Read the model definition and answer for the solid it produces. Units are mm, in the model's axes. Face numbers are marked on the shaded views. Round coordinates to 2 decimals unless told otherwise and drop trailing zeros. Loops run counter-clockwise (first coordinate to the right, second up) from the corner with the lowest first, then second, coordinate; pieces in that order, holes last. Notation, with made-up numbers: (12.25, 83.5) - (45.25, 83.5) arc R11 ccw to (45.25, 92.5) - close; hole circle Ø2 at (56, 24.5). An arc over 180 degrees is marked (long way). Use CSV: the item, a comma, the result in double quotes. Start each with the question number.
1. Find section C-C (z = 21.25). Give the vertices of the cut face in (x, y), and give its area (3 significant figures).
2. Consider line 1 along Y through (x, z) = (0, 22.75); line 2 along X through (y, z) = (1.25, 28.25). Determine where each line is inside the solid, lowest interval first.
3. Determine the mould class of the marked faces 1, 2 and 3 for opening direction X: +X half, -X half, draft (parallel to the pull), parting line (faces both ways), or undercut.
4. Find section A-A (y = 0). Give the vertices of the cut face in (x, z), and give its area (3 significant figures).
5. Find section D-D (z = 17). Give the vertices of the cut face in (x, y).
6. Given pin 1 Ø1 at (y, z) = (-1, 6.5) entering from +X; pin 2 Ø5 at (x, z) = (-0.5, 16.5) entering from +Y; pin 3 Ø2 at (x, z) = (-1.5, 15.5) entering from +Y, each flat-ended and moving along its own axis, determine where each tip first touches the part or whether it passes through.
from build123d import *

# Parameters (mm, degrees)
SKETCH1_R           = 4.5
SKETCH1_R_2         = 2.5
BOSS_EXTRUDE1_DEPTH = 2
SKETCH5_R           = 2.5
BOSS_EXTRUDE3_DEPTH = 28
SKETCH6_R           = 1.5
CUT_EXTRUDE3_DEPTH  = 10
BOSS_EXTRUDE4_START = 1
SKETCH7_R           = 2.5
BOSS_EXTRUDE4_DEPTH = 1
FILLET1_R           = 2


with BuildPart() as part:
    # Sketch1 → Boss-Extrude1 (new body)
    with BuildSketch(Plane.XY):
        Circle(SKETCH1_R)
        Circle(SKETCH1_R_2, mode=Mode.SUBTRACT)
    extrude(amount=BOSS_EXTRUDE1_DEPTH)



with BuildPart() as body_2:
    # Sketch5 → Boss-Extrude3 (new body)
    with BuildSketch(Plane.XY.offset(2)):
        Circle(SKETCH5_R)
    extrude(amount=BOSS_EXTRUDE3_DEPTH)

    # Sketch6 → Cut-Extrude3 (cut)
    with BuildSketch(Plane.XY.offset(30)):
        Circle(SKETCH6_R)
    extrude(amount=-CUT_EXTRUDE3_DEPTH, mode=Mode.SUBTRACT)


with BuildPart() as part_1:
    add(part.part)

    add(body_2.part)  # Boss-Extrude4 merges body 2
    # Sketch7 → Boss-Extrude4 (add)
    with BuildSketch(Plane(origin=(0, 0, 2), x_dir=(-1, 0, 0), z_dir=(0, 0, -1)).offset(BOSS_EXTRUDE4_START)):
        Circle(SKETCH7_R)
    extrude(amount=-BOSS_EXTRUDE4_DEPTH)

    # Fillet1
    # the kernel refuses this fillet: 2 mm, written as the material it takes off along each edge
    with BuildSketch(Plane(origin=(0, 0, 0), x_dir=(1, 0, 0), z_dir=(0, -1, 0))) as fillet1_piece_1:
        with BuildLine():
            CenterArc((4.232050808, 2), FILLET1_R, 210, 60)
            Line((2.5, 1), (2.465358984, 0.98))
            ThreePointArc((2.465358984, 0.98), (2.46, 0.5), (2.46, 0))
            Line((2.46, 0), (2.5, -0.04))
            Line((2.5, -0.04), (4.232050808, -0.04))
            Line((4.232050808, -0.04), (4.232050808, 0))
        make_face()
    revolve(axis=Axis((0, 0, 0), (0, 0, 1)), mode=Mode.SUBTRACT)


solid = part_1.part
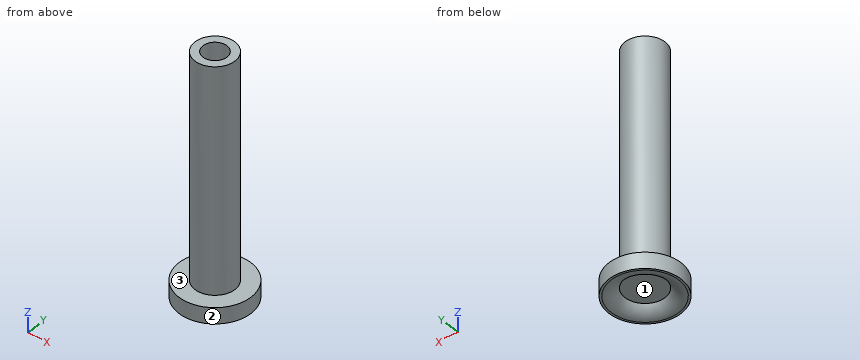
Filled sheet:
1,outline,"circle Ø5 at (0, 0); hole circle Ø3 at (0, 0)"
1,area,"12.6 mm²"
2,line 1,"y = -2.5 to -1.5, 1.5 to 2.5"
2,line 2,"x = -2.17 to -0.83, 0.83 to 2.17"
3,face 1,"undercut"
3,face 2,"parting line"
3,face 3,"draft"
4,outline,"(-4.5, 0) - (-4.23, 0) arc R2 ccw to (-2.5, 1) - (2.5, 1) arc R2 ccw to (4.23, 0) - (4.5, 0) - (4.5, 2) - (2.5, 2) - (2.5, 30) - (1.5, 30) - (1.5, 20) - (-1.5, 20) - (-1.5, 30) - (-2.5, 30) - (-2.5, 2) - (-4.5, 2) - close"
4,area,"122 mm²"
5,outline,"circle Ø5 at (0, 0)"
6,pin 1,"stops at x = 2.45"
6,pin 2,"stops at y = 2.5"
6,pin 3,"stops at y = 2.45"
